Job drawing, mm, ordinate dimensions from the low corner. One solid piece. A direction names the side the tool comes from. Give positions to 0.01 mm unless a question says otherwise; leave off trailing zeros. Loops run counter-clockwise (first coordinate to the right, second up) from the corner with the lowest first, then second, coordinate; pieces in that order, holes last. Notation, with made-up numbers: (15, 78) -> (30, 78) arc R19 ccw to (30, 113) -> close; hole circle Ø1 at (78.5, 30). An arc over 180 degrees is marked (long way). Answer as a JSON object with one key per item and string values. Group by question number.
Q1. Band-saw the part on B-B, the plane y = 2.5. Write the cut outline in (x, z), plus the area to 3 significant figures.
Q2. Wall check: probe 1 along X at (y, z) = (6, 4.5); probe 2 along Z at (x, y) = (4, 1.1); probe 3 along X at (y, z) = (1, 9.25). Give the ranges that are in metal, low to high. Write a range as from..to.
Q3. Tool access for the marked faces 1, 2 and 3: list every direction of +Z, -Z, +X, -X, +Y, -Y with a clear straight run to the whole face (end or side of a thin tool).
Q4. Drop flat-ended pins along their axis: pin 1 (3 mm diameter, centred on x = 5, z = 8, fed in from +Y); pin 2 (3.5 mm diameter, centred on y = 7.5, z = 7.5, fed in from +X); pin 3 (1.8 mm diameter, centred on x = 25.5, z = 8, fed in from +Y). Give the stop position or say it passes through.
Q5. Band-saw the part on A-A, the plane z = 7.5. Count the separate pieces of the cut face and the enclosed holes in it, plus the area to 3 significant figures.
Q6. Band-saw the part on D-D, the plane y = 7.5. Write the cut outline in (x, z), plus the area to 3 significant figures.
Q7. Two-plate mould, pull along Z, no slides. Class the marked faces 4, 5 and 6: pulls with the +Z half, pulls with the -Z half, needs draft (parallel to the pull), parting line crosses it, or undercut.
Q8. Band-saw the part on C-C, the plane x = 26. Write the cut outline in (y, z), plus the area to 3 significant figures.
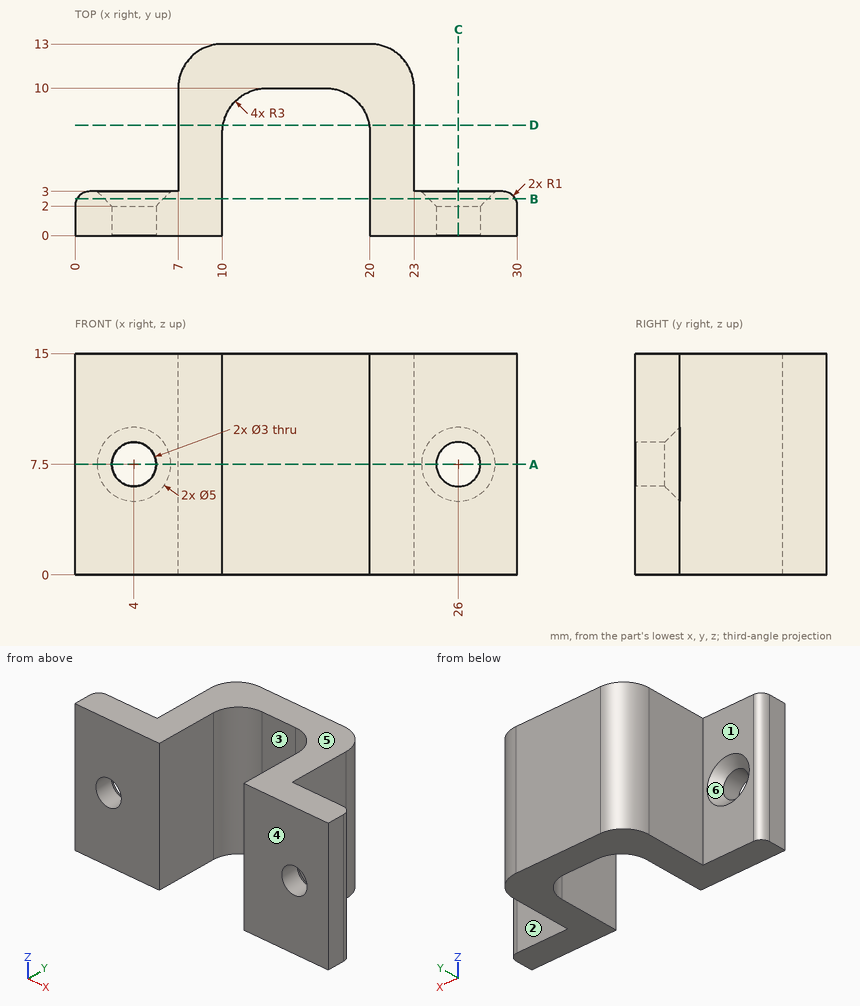
Worked answers:
{
 "1": {"outline": "(0.13, 0) -> (10, 0) -> (10, 15) -> (0.13, 15) -> close; (20, 0) -> (29.87, 0) -> (29.87, 15) -> (20, 15) -> close; hole circle Ø4 at (4, 7.5); hole circle Ø4 at (26, 7.5)", "area": "271 mm2"},
 "2": {"probe 1": "7..10, 20..23", "probe 2": "0..6, 9..15", "probe 3": "0..10, 20..30"},
 "3": {"face 1": "+Z, -Z, -X, +Y", "face 2": "+Z, -Z, +X, +Y", "face 3": "+Z, -Z, -Y"},
 "4": {"pin 1": "y = 3", "pin 2": "x = 23", "pin 3": "y = 2.11"},
 "5": {"separate pieces": "3", "enclosed holes": "0", "area": "130 mm2"},
 "6": {"outline": "(7, 0) -> (10.04, 0) -> (10.04, 15) -> (7, 15) -> close; (19.96, 0) -> (23, 0) -> (23, 15) -> (19.96, 15) -> close", "area": "91.3 mm2"},
 "7": {"face 4": "needs draft", "face 5": "pulls with the +Z half", "face 6": "undercut"},
 "8": {"outline": "(0, 0) -> (3, 0) -> (3, 5) -> (2, 6) -> (0, 6) -> close; (0, 9) -> (2, 9) -> (3, 10) -> (3, 15) -> (0, 15) -> close", "area": "35.0 mm2"}
}
